Geometry check sheet. Reference: the model listing, model coordinates, mm. A direction names the side the tool comes from. Coordinates: 2 decimals unless noted, no trailing zeros. Loops run counter-clockwise (first coordinate to the right, second up) from the corner with the lowest first, then second, coordinate; pieces in that order, holes last. Notation, with made-up numbers: (19.25, 15) - (43.25, 15) arc R18 cw to (43.25, 34) - close; hole circle Ø7 at (49, 21). An arc over 180 degrees is marked (long way). One line per item, written item: value.
Autodesk Inventor part; units mm, degrees
ref_plane "YZ Plane" through (0, 0, 0) normal (1, 0, 0) x (0, 1, 0)
ref_plane "XZ Plane" through (0, 0, 0) normal (0, 1, 0) x (-1, 0, 0)
ref_plane "XY Plane" through (0, 0, 0) normal (0, 0, 1) x (1, 0, 0)
sketch "Szkic1" plane through (0, 0, 0) normal (1, 0, 0) x (0, 1, 0)
  line L0 (-37, 37) -> (37, 37)
  line L1 (37, 37) -> (37, -37)
  line L2 (37, -37) -> (-37, -37)
  line L3 (-37, -37) -> (-37, 37)
  line L4 (-37, 37) -> (37, -37) construction
  line L5 (37, 37) -> (-37, -37) construction
  point P0 (0, 0)
  dimension "d0" = 74
  dimension "d1" = 74
extrude "Wyciągnięcie proste1" add sketch "Szkic1" along normal blind 18
sketch "Szkic2" plane through (18, 0, 0) normal (1, 0, 0) x (0, 0, -1)
  circle A0 centre (-27.4, 31) radius 2.85
  line L0 (37, 37) -> (-37, 37)
  line L1 (-37, 37) -> (-37, -37)
  circle A1 centre (-27.4, 0) radius 2.85
  circle A2 centre (-27.4, -31) radius 2.85
  circle A3 centre (27.4, 31) radius 2.85
  line L2 (37, -37) -> (37, 37)
  circle A4 centre (27.4, 0) radius 2.85
  circle A5 centre (27.4, -31) radius 2.85
  line L3 (-29.8537, 35.25) -> (-24.9463, 35.25)
  line L4 (-24.9463, 35.25) -> (-22.4925, 31)
  line L5 (-22.4925, 31) -> (-24.9463, 26.75)
  line L6 (-24.9463, 26.75) -> (-29.8537, 26.75)
  line L7 (-29.8537, 26.75) -> (-32.3075, 31)
  line L8 (-32.3075, 31) -> (-29.8537, 35.25)
  line L9 (-29.8537, 4.25) -> (-24.9463, 4.25)
  line L10 (-24.9463, 4.25) -> (-22.4925, 0)
  line L11 (-22.4925, 0) -> (-24.9463, -4.25)
  line L12 (-24.9463, -4.25) -> (-29.8537, -4.25)
  line L13 (-29.8537, -4.25) -> (-32.3075, 0)
  line L14 (-32.3075, 0) -> (-29.8537, 4.25)
  line L15 (-29.8537, -26.75) -> (-24.9463, -26.75)
  line L16 (-24.9463, -26.75) -> (-22.4925, -31)
  line L17 (-22.4925, -31) -> (-24.9463, -35.25)
  line L18 (-24.9463, -35.25) -> (-29.8537, -35.25)
  line L19 (-29.8537, -35.25) -> (-32.3075, -31)
  line L20 (-32.3075, -31) -> (-29.8537, -26.75)
  line L21 (29.8537, 35.25) -> (32.3075, 31)
  line L22 (32.3075, 31) -> (29.8537, 26.75)
  line L23 (29.8537, 26.75) -> (24.9463, 26.75)
  line L24 (24.9463, 26.75) -> (22.4925, 31)
  line L25 (22.4925, 31) -> (24.9463, 35.25)
  line L26 (24.9463, 35.25) -> (29.8537, 35.25)
  line L27 (29.8537, 4.25) -> (32.3075, 0)
  line L28 (32.3075, 0) -> (29.8537, -4.25)
  line L29 (29.8537, -4.25) -> (24.9463, -4.25)
  line L30 (24.9463, -4.25) -> (22.4925, 0)
  line L31 (22.4925, 0) -> (24.9463, 4.25)
  line L32 (24.9463, 4.25) -> (29.8537, 4.25)
  line L33 (29.8537, -26.75) -> (32.3075, -31)
  line L34 (32.3075, -31) -> (29.8537, -35.25)
  line L35 (29.8537, -35.25) -> (24.9463, -35.25)
  line L36 (24.9463, -35.25) -> (22.4925, -31)
  line L37 (22.4925, -31) -> (24.9463, -26.75)
  line L38 (24.9463, -26.75) -> (29.8537, -26.75)
  point P0 (0, 0)
  point P1 (27.4, -26.75)
  dimension "d4" = 6
  dimension "d5" = 5.7
  dimension "d6" = 9.6
  dimension "d7" = 31
  dimension "d8" = 31
  dimension "d9" = 5.7
  dimension "d10" = 5.7
  dimension "d11" = 9.6
  dimension "d12" = 5.7
  dimension "d13" = 5.7
  dimension "d14" = 5.7
  dimension "d15" = 8.5
  dimension "d16" = 8.5
  dimension "d17" = 8.5
  dimension "d18" = 8.5
  dimension "d19" = 8.5
  dimension "d20" = 8.5
extrude "Wyciągnięcie proste2" cut sketch "Szkic2" against normal through all contours A0 | A1 | A2 | A3 | A4 | A5
extrude "Wyciągnięcie proste3" cut sketch "Szkic2" against normal blind 10 contours A0 | A1 | A2 | A3 | A4 | A5 | L3 L4 L5 L6 L7 L8 | L9 L10 L11 L12 L13 L14 | L15 L16 L17 L18 L19 L20 | L21 L22 L23 L24 L25 L26 | L27 L28 L29 L30 L31 L32 | L33 L34 L35 L36 L37 L38
sketch "Szkic3" plane through (0, -37, 37) normal (0, 0, 1) x (1, 0, 0)
  line L0 (0, 0) -> (0, 74)
  line L1 (0, 72.5) -> (2, 72.5)
  line L2 (2, 72.5) -> (2, 63.5)
  line L3 (2, 63.5) -> (0, 63.5)
  line L4 (0, 63.5) -> (0, 72.5)
  line L5 (0, 74) -> (18, 74)
  line L6 (0, 10.5) -> (2, 10.5)
  line L7 (2, 10.5) -> (2, 1.5)
  line L8 (2, 1.5) -> (0, 1.5)
  line L9 (0, 1.5) -> (0, 10.5)
  point P0 (0, 37)
  point P1 (0, 1.5)
  point P2 (0, 63.5)
  dimension "d25" = 1.5
  dimension "d26" = 9
  dimension "d27" = 2
  dimension "d28" = 2
  dimension "d29" = 9
  dimension "d30" = 1.5
extrude "Wyciągnięcie proste4" cut sketch "Szkic3" against normal through all
sketch "Szkic4" plane through (0, -37, 37) normal (0, 0, 1) x (1, 0, 0)
  line L0 (10.5, 60.5) -> (10.5, 44.5)
  line L1 (10.5, 44.5) -> (16.3, 44.5)
  line L2 (16.3, 44.5) -> (16.3, 50.5)
  line L3 (16.3, 60.5) -> (10.5, 60.5)
  line L4 (16.3, 50.5) -> (18, 50.5)
  line L5 (18, 50.5) -> (18, 54.5)
  line L6 (18, 54.5) -> (16.3, 54.5)
  line L7 (16.3, 54.5) -> (16.3, 60.5)
  line L8 (16.3, 50.5) -> (16.3, 54.5) construction
  line L9 (18, 74) -> (18, 0)
  line L10 (18, 63.75) -> (8, 63.75)
  line L11 (18, 63.75) -> (8, 63.75)
  point P0 (0, 37)
  dimension "d33" = 5.8
  dimension "d34" = 4
  dimension "d35" = 1.7
  dimension "d36" = 6
  dimension "d37" = 16
  dimension "d38" = 3.25
extrude "Wyciągnięcie proste5" cut sketch "Szkic4" against normal blind 20
properties part number "XItemEndCoverConnector" material "Tworzywo sztuczne ABS"
(1) Cross-section at A-A on y = 32. Record the cut outline in (x, z).
Reply:
outline: (2, -37) - (18, -37) - (18, -31.73) - (8, -31.73) - (8, -30.07) - (2, -30.07) - close; (2, -24.73) - (8, -24.73) - (8, -23.07) - (18, -23.07) - (18, 23.07) - (8, 23.07) - (8, 24.73) - (2, 24.73) - close; (2, 30.07) - (8, 30.07) - (8, 31.73) - (18, 31.73) - (18, 37) - (2, 37) - close
(2) Access from +Z, -Z, +X, -X, +Y, -Y to the whole of each face (thin tool, end or side, straight path). Record for faces 1 (the face through (4.056, 0.125, 30.247)), 2 (the face through (2, 31, 1)), 3 (the face through (13.07, 28.905, 23.702)).
Reply:
face 1: +X, -X
face 2: +Z, -Z, -X
face 3: +X
(3) Go/stop test with flat-tipped pins: pin 1 Ø5 at (y, z) = (0, 27.4) entering from +X; pin 2 Ø7 at (y, z) = (31, 28) entering from +X. Record where each tip stops, or that it passes through.
Reply:
pin 1: through
pin 2: x = 8
(4) Cross-section at C-C on x = 12. State how many separate pieces and enclosed holes the cut face has, and give its area (3 significant figures).
Reply:
separate pieces: 1
enclosed holes: 6
area: 4,780 mm2
(5) Cross-section at B-B on z = -11. Record the cut outline in (x, y).
Reply:
outline: (0, -37) - (18, -37) - (18, 37) - (0, 37) - (0, 35.5) - (2, 35.5) - (2, 26.5) - (0, 26.5) - (0, -26.5) - (2, -26.5) - (2, -35.5) - (0, -35.5) - close
(6) Release check for a two-part mould opening along Y. For faces 4 (the face through (13.07, 33.095, -23.702)), 5 (the face through (9, -1, 37)) record: pulls with the +Y half, pulls with the -Y half, needs draft (parallel to the pull), parting line crosses it, or undercut.
Reply:
face 4: undercut
face 5: needs draft
(7) Material ranges on probe 1 along Y at (x, z) = (3.3, 27.4); probe 2 along Z at (x, y) = (16.25, -31); probe 3 along Y at (x, z) = (9.25, 25.5), recorded low to high. Write a range as from..to.
Reply:
probe 1: -37..-33.85, -28.15..-2.85, 2.85..28.15, 33.85..37
probe 2: -37..-32.31, -22.49..22.49, 32.31..37
probe 3: -37..-35.25, -26.75..-4.25, 4.25..26.75, 35.25..37
